Check sheet for the modelled part. Datum: model origin and axes. Units: mm. Coordinates: 2 decimals unless noted, no trailing zeros. Order: outer loops, then holes, each group sorted by start corner. A loop starts at its lowest first (then second) coordinate and runs counter-clockwise, first axis right, second up. Notation, with made-up numbers: (32.25, 86) -> (61.25, 86) arc R12 ccw to (61.25, 104) -> close; hole circle Ø1 at (-18, 15.5). An arc over 180 degrees is marked (long way). Put each result on its own line as item: value. Start each with the question number.
```python
from build123d import *

# Parameters (mm, degrees)
SKETCH1_R           = 3.3782
BOSS_EXTRUDE1_DEPTH = 5.588


with BuildPart() as part:
    # Sketch1 (on Top Plane) → Boss-Extrude1 (new body)
    with BuildSketch(Plane(origin=(0, 0, 0), x_dir=(1, 0, 0), z_dir=(0, 1, 0))):
        Polygon((0, 0), (0, 469.9), (439.7375, 469.9), (439.7375, 773.938), (994.205378114, 773.938), (885.3805, 697.738), (885.3805, 495.45319999), (177.8, 0), align=None)
        with Locations(Location((24.6253, 21.463, 0), (0, 0, 270))):
            Circle(SKETCH1_R, mode=Mode.SUBTRACT)
        with Locations(Location((69.0753, 323.85, 0), (0, 0, 270))):
            Circle(SKETCH1_R, mode=Mode.SUBTRACT)
        with Locations(Location((495.8715, 438.15, 0), (0, 0, 270))):
            Circle(SKETCH1_R, mode=Mode.SUBTRACT)
        with Locations(Location((495.8715, 640.588, 0), (0, 0, 270))):
            Circle(SKETCH1_R, mode=Mode.SUBTRACT)
        with Locations(Location((829.2465, 640.588, 0), (0, 0, 270))):
            Circle(SKETCH1_R, mode=Mode.SUBTRACT)
    extrude(amount=BOSS_EXTRUDE1_DEPTH)


solid = part.part
```
1) Sectioned sample at C-C (x = 603.5). Record the boundary of the cut face in (y, z).
2) Gauge pin test, flat ends, axial feed: pin 1 (4 mm diameter, centred on x = 24.63, z = -21.46, fed in from +Y); pin 2 (3 mm diameter, centred on y = 2.5, z = -690, fed in from -X); pin 3 (3 mm diameter, centred on x = 668, y = 1, fed in from +Z). Record the tip position at first contact, or that the pin passes through.
3) Scan lines: line 1 along X through (y, z) = (2.6, -438.15); line 2 along Z through (x, y) = (113, 0.35); line 3 along X through (y, z) = (3.7, -537). Record each from-to range of solid material in increasing order. Write a range as [from, to].
4) Sectioned sample at A-A (y = 3). Record the boundary of the cut face in (x, z), plus the area to 3 significant figures.
5) Sectioned sample at B-B (z = -584). Record the boundary of the cut face in (x, y), plus the area to 3 significant figures.
Entries:
1. outline: (0, -773.94) -> (5.59, -773.94) -> (5.59, -298.08) -> (0, -298.08) -> close
2. pin 1: passes through
2. pin 2: stops at x = 439.74
2. pin 3: stops at z = -342.19
3. line 1: x = [0, 492.49], [499.25, 803.54]
3. line 2: z = [-469.9, 0]
3. line 3: x = [439.74, 885.38]
4. outline: (0, -469.9) -> (439.74, -469.9) -> (439.74, -773.94) -> (994.21, -773.94) -> (885.38, -697.74) -> (885.38, -495.45) -> (177.8, 0) -> (0, 0) -> close; hole circle Ø6.76 at (24.63, -21.46); hole circle Ø6.76 at (69.08, -323.85); hole circle Ø6.76 at (495.87, -640.59); hole circle Ø6.76 at (495.87, -438.15); hole circle Ø6.76 at (829.25, -640.59)
4. area: 380,000 mm2
5. outline: (439.74, 0) -> (885.38, 0) -> (885.38, 5.59) -> (439.74, 5.59) -> close
5. area: 2,490 mm2
